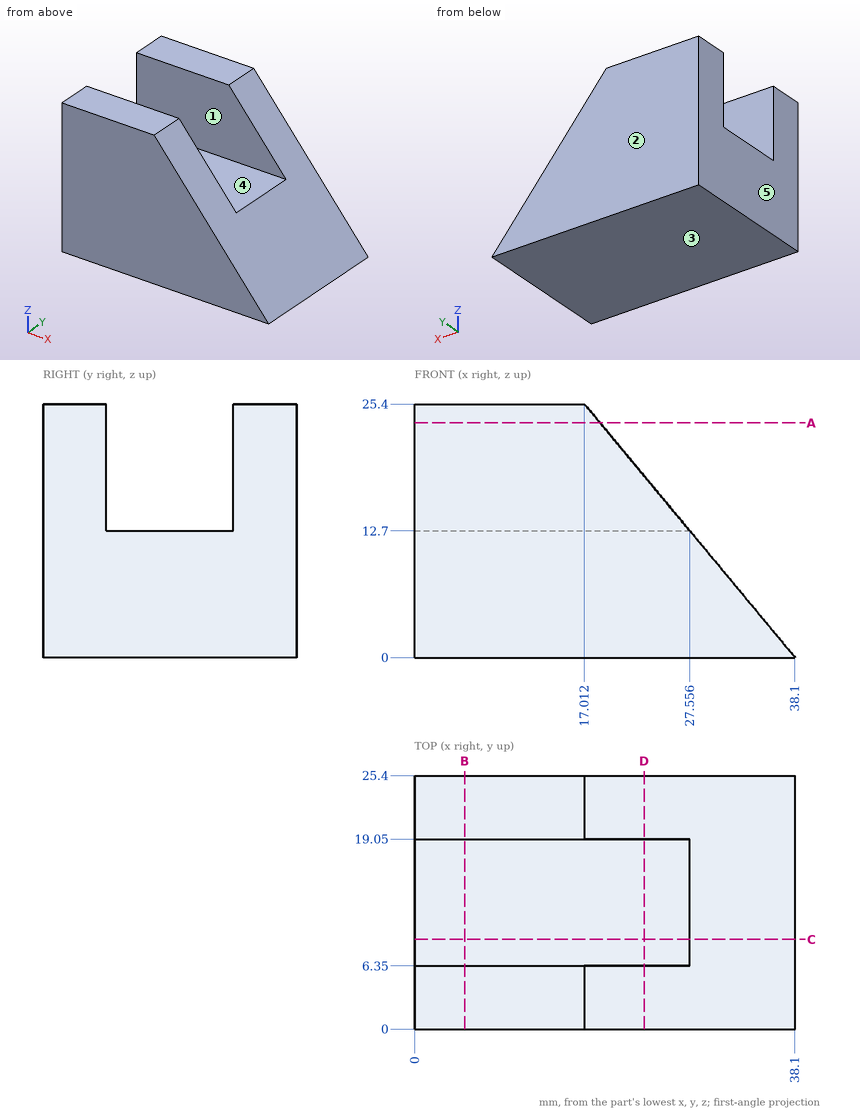
Geometry: see drawing. Coordinates: mm, zero at the bounding-box minimum. A direction names the side the tool comes from. Round coordinates to 2 decimals unless told otherwise and drop trailing zeros. Write each loop counter-clockwise with the first axis right and the second up, starting at its lowest first coordinate (ties: lowest second). Pieces come first, ordered by that corner, then holes. Notation, with made-up numbers: M 51.25,-13.75 L 80.25,-13.75 A13 cw 80.25,-0.75 Z; hole C -33,20 d5. An arc over 180 degrees is marked long. Answer as a JSON object with one key per item and string values. Group by question number.
(1) Mould query, pull axis Y, two halves, no side actions, for the marked faces 1, 2 and 3. Classes: +Y half, -Y half, draft (parallel to the pull), parting line (faces both ways), or undercut.
(2) Reachability of the marked faces 4 and 5 from +Z, -Z, +X, -X, +Y, -Y: full face, straight path, thin tool, end or side. Return the list, or none.
(3) First-contact query: pin 1 (3 mm diameter, centred on y = 15, z = 7.5, fed in from +X); pin 2 (6 mm diameter, centred on y = 19, z = 7.5, fed in from +X); pin 3 (6.5 mm diameter, centred on x = 13, y = 14, fed in from +Z). Flat tips, straight axial feed; report the tip coordinate or a pass-through.
(4) Ray query, line 1 (Z direction, x = 23, y = 15); line 2 (Y direction, x = 20, z = 20.5); line 3 (X direction, y = 20.25, z = 11.5). Return the intervals inside material, ascending. Write a range as [from, to].
(5) Section query D-D on x = 23. Output: boundary loops of the cut face in (y, z).
(6) Section query A-A on z = 23.5. Output: boundary loops of the cut face in (x, y), then the cut area to 3 significant figures.
(7) Section query C-C on y = 9. Output: boundary loops of the cut face in (x, z), then the cut area to 3 significant figures.
(8) Section query B-B on x = 5. Output: boundary loops of the cut face in (y, z).
Computed values:
{
 "1": {"face 1": "undercut", "face 2": "+Y half", "face 3": "draft"},
 "2": {"face 4": "+Z, +X, -X", "face 5": "+Z, -Z, -X, +Y, -Y"},
 "3": {"pin 1": "x = 33.12", "pin 2": "x = 34.36", "pin 3": "z = 12.7"},
 "4": {"line 1": "[0, 12.7]", "line 2": "[0, 6.35], [19.05, 25.4]", "line 3": "[0, 28.55]"},
 "5": {"outline": "M 0,0 L 25.4,0 L 25.4,18.19 L 19.05,18.19 L 19.05,12.7 L 6.35,12.7 L 6.35,18.19 L 0,18.19 Z"},
 "6": {"outline": "M 0,0 L 18.59,0 L 18.59,6.35 L 0,6.35 Z; M 0,19.05 L 18.59,19.05 L 18.59,25.4 L 0,25.4 Z", "area": "236 mm^2"},
 "7": {"outline": "M 0,0 L 38.1,0 L 27.56,12.7 L 0,12.7 Z", "area": "417 mm^2"},
 "8": {"outline": "M 0,0 L 25.4,0 L 25.4,25.4 L 19.05,25.4 L 19.05,12.7 L 6.35,12.7 L 6.35,25.4 L 0,25.4 Z"}
}
